Geometry check sheet. Reference: the model listing, model coordinates, mm. Face numbers are marked on the shaded views. A direction names the side the tool comes from. Give positions to 0.01 mm unless a question says otherwise; leave off trailing zeros. Order: outer loops, then holes, each group sorted by start corner. A loop starts at its lowest first (then second) coordinate and runs counter-clockwise, first axis right, second up.
```python
from build123d import *

# Parameters (mm, degrees)
SKETCH1_W           = 19.05
SKETCH1_H           = 19.36
SKETCH1_R           = 2.5527
SKETCH1_H_2         = 7
BOSS_EXTRUDE1_DEPTH = 6
SKETCH3_W           = 19.05
SKETCH3_H           = 7
BOSS_EXTRUDE2_DEPTH = 45
SKETCH4_R           = 2.6
CUT_EXTRUDE1_DEPTH  = 27.36


with BuildPart() as part:
    # Sketch1 → Boss-Extrude1 (new body)
    with BuildSketch(Plane.XY):
        with Locations((0, 13.18)):
            Rectangle(SKETCH1_W, SKETCH1_H)
        with Locations((0, 16.51)):
            Circle(SKETCH1_R, mode=Mode.SUBTRACT)
        with Locations((0, -13.18)):
            Rectangle(SKETCH1_W, SKETCH1_H)
        with Locations((0, -16.51)):
            Circle(SKETCH1_R, mode=Mode.SUBTRACT)
        Rectangle(SKETCH1_W, SKETCH1_H_2)
    extrude(amount=-BOSS_EXTRUDE1_DEPTH)

    # Sketch3 → Boss-Extrude2 (add)
    with BuildSketch(Plane.XY):
        Rectangle(SKETCH3_W, SKETCH3_H)
    extrude(amount=-BOSS_EXTRUDE2_DEPTH)

    # Sketch4 → Cut-Extrude1 (cut, through all)
    with BuildSketch(Plane(origin=(0, 3.5, 0), x_dir=(1, 0, 0), z_dir=(0, 1, 0))):
        with Locations((0, 28.15)):
            Circle(SKETCH4_R)
    extrude(amount=-CUT_EXTRUDE1_DEPTH, mode=Mode.SUBTRACT)


solid = part.part
```
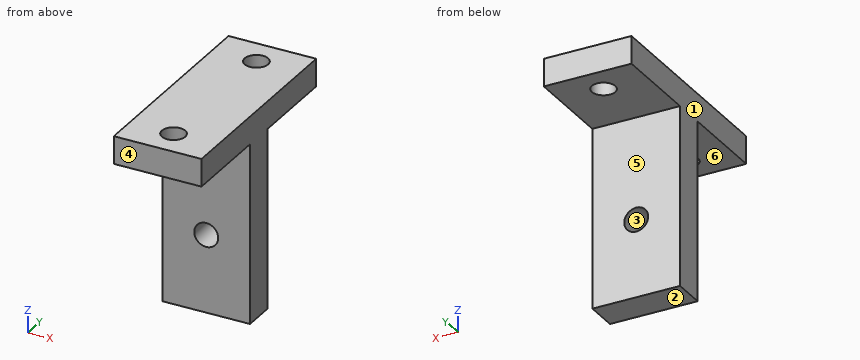
Q1. Thickness scan on L1, parallel to Y at x = 0, z = -4.2; L2, parallel to X at y = 0, z = -28 (3 decimals); L3, parallel to Z at x = 0, y = 0.25. Record the ranges inside material, lowest first.
Q2. Cross-section at B-B, the plane y = 16.51. Record the boundary of the cut face in (x, z) (3 decimals).
Q3. Cross-section at C-C, the plane z = -28.15. Record the boundary of the cut face in (x, y) (3 decimals), and give its area (4 significant figures).
Q4. Cross-section at D-D, the plane x = -8. Record the boundary of the cut face in (y, z).
Q5. Access from +Z, -Z, +X, -X, +Y, -Y to the whole of each face (thin tool, end or side, straight path). Record for the marked faces 4, 5 and 6.
Q6. Release check for a two-part mould opening along X. For the marked faces 1, 2 and 3 record: pulls with the +X half, pulls with the -X half, needs draft (parallel to the pull), parting line crosses it, or undercut.
Q7. Cross-section at A-A, the plane x = 0. Record the boundary of the cut face in (y, z).
Q8. Gauge pin test, flat ends, axial feed: P1, Ø4, axis at x = -4.5, z = -33, coming from the -Y side; P2, Ø8, axis at x = 0, y = -16.51, coming from the -Z side; P3, Ø9.5, axis at x = -1.5, z = -19, coming from the +Y side; P4, Ø12, axis at y = -11, z = -25.5, coming from the -X side. Record the tip position at first contact, or that the pin passes through.
Answers follow:
1. L1: y = -22.86 to -19.06, -13.96 to 13.96, 19.06 to 22.86
1. L2: x = -9.525 to -2.596, 2.596 to 9.525
1. L3: z = -45 to -30.75, -25.55 to 0
2. outline: (-9.525, -6) - (-2.553, -6) - (-2.553, 0) - (-9.525, 0) - close; (2.553, -6) - (9.525, -6) - (9.525, 0) - (2.553, 0) - close
3. outline: (-9.525, -3.5) - (-2.6, -3.5) - (-2.6, 3.5) - (-9.525, 3.5) - close; (2.6, -3.5) - (9.525, -3.5) - (9.525, 3.5) - (2.6, 3.5) - close
3. area: 96.95 mm2
4. outline: (-22.86, -6) - (-3.5, -6) - (-3.5, -45) - (3.5, -45) - (3.5, -6) - (22.86, -6) - (22.86, 0) - (-22.86, 0) - close
5. face 4: +Z, -Z, +X, -X, -Y
5. face 5: -Z, +X, -X, +Y
5. face 6: -Z, +X, -X, -Y
6. face 1: pulls with the -X half
6. face 2: needs draft
6. face 3: undercut
7. outline: (-22.86, -6) - (-19.06, -6) - (-19.06, 0) - (-22.86, 0) - close; (-13.96, -6) - (-3.5, -6) - (-3.5, -25.55) - (3.5, -25.55) - (3.5, -6) - (13.96, -6) - (13.96, 0) - (-13.96, 0) - close; (-3.5, -45) - (3.5, -45) - (3.5, -30.75) - (-3.5, -30.75) - close; (19.06, -6) - (22.86, -6) - (22.86, 0) - (19.06, 0) - close
8. P1: stops at y = -3.5
8. P2: stops at z = -6
8. P3: stops at y = 3.5
8. P4: passes through
